Design review of the part built by this model. Coordinates are the model's own, in mm. Face numbers are marked on the shaded views. A direction names the side the tool comes from. Coordinates: 2 decimals unless noted, no trailing zeros. Write each loop counter-clockwise with the first axis right and the second up, starting at its lowest first coordinate (ties: lowest second). Pieces come first, ordered by that corner, then holes. Notation, with made-up numbers: (-28, 47) -> (22, 47) arc R15 ccw to (22, 69) -> close; hole circle Ø7 at (13, -22.5). An arc over 180 degrees is marked (long way). Write item = value, one per line. Start each with the question number.
Autodesk Inventor part; units mm, degrees
ref_plane "YZ Plane" through (0, 0, 0) normal (1, 0, 0) x (0, 1, 0)
ref_plane "XZ Plane" through (0, 0, 0) normal (0, 1, 0) x (-1, 0, 0)
ref_plane "XY Plane" through (0, 0, 0) normal (0, 0, 1) x (1, 0, 0)
sketch "Boceto3" plane through (0, 0, 0) normal (0, 0, 1) x (1, 0, 0)
  line L0 (-30, 8) -> (-30, -12)
  line L1 (-30, -22) -> (30, -22)
  line L2 (30, -12) -> (30, 8)
  arc A0 (-19.4936, 8) -> (19.4936, 8) centre (0, 22) ccw
  line L3 (-30, 8) -> (-19.4936, 8)
  line L4 (19.4936, 8) -> (30, 8)
  line L5 (-30, -22) -> (-70, -22)
  line L6 (-70, -22) -> (-70, -12)
  line L7 (-70, -12) -> (-30, -12)
  line L8 (30, -22) -> (70, -22)
  line L9 (70, -22) -> (70, -12)
  line L10 (70, -12) -> (30, -12)
  point P0 (0, 0)
  point P1 (0, -22)
  point P2 (30, 0)
  dimension "d16" = 60
  dimension "d38" = 24
  dimension "d39" = 10.5064
  dimension "d40" = 10.5064
  dimension "d41" = 30
  dimension "d42" = 30
  dimension "d43" = 22
  dimension "d44" = 40
  dimension "d45" = 10
  dimension "d46" = 40
  dimension "d47" = 10
extrude "Extrusión2" add sketch "Boceto3" along normal blind 9
sketch "Boceto5" plane through (0, 0, 9) normal (0, 0, 1) x (1, 0, 0)
  line L0 (-70, -22) -> (70, -22)
  line L1 (70, -22) -> (70, -12)
  line L2 (70, -12) -> (30, -12)
  line L3 (30, -12) -> (30, 8)
  line L4 (30, 8) -> (19.4936, 8)
  arc A0 (-19.4936, 8) -> (19.4936, 8) centre (0, 22) ccw
  line L5 (-19.4936, 8) -> (-30, 8)
  line L6 (-30, 8) -> (-30, -12)
  line L7 (-30, -12) -> (-70, -12)
  line L8 (-70, -12) -> (-70, -22)
  point P0 (0, 0)
  point P1 (-52.5, -17)
  point P2 (52.5, -17)
  dimension "d55" = 5
  dimension "d56" = 17.5
  dimension "d57" = 5
  dimension "d58" = 17.5
hole "Agujero2" at (-52.5, -17, 9) at (52.5, -17, 9) direction (0, 0, -1) diameter 5 depth 10 tip angle 118
sketch "Boceto6" plane through (-70, -22, 0) normal (0, -1, 0) x (1, 0, 0)
  line L0 (0, 0) -> (140, 0)
  line L1 (140, 0) -> (140, 9)
  line L2 (0, 9) -> (140, 9)
  line L3 (0, 0) -> (0, 9)
  line L4 (40, 0) -> (40, 9)
  line L5 (100, 0) -> (100, 9)
  point P0 (70, 0)
  point P1 (47.5, 4.5)
  point P2 (92.5, 4.5)
  dimension "d67" = 47.5
  dimension "d68" = 47.5
  dimension "d69" = 4.5
  dimension "d70" = 4.5
hole "Agujero3" at (-22.5, -22, 4.5) at (22.5, -22, 4.5) direction (0, 1, 0) diameter 5 depth 20 tip angle 118
properties part number "Soporte para Motor 2" material "Abedul"
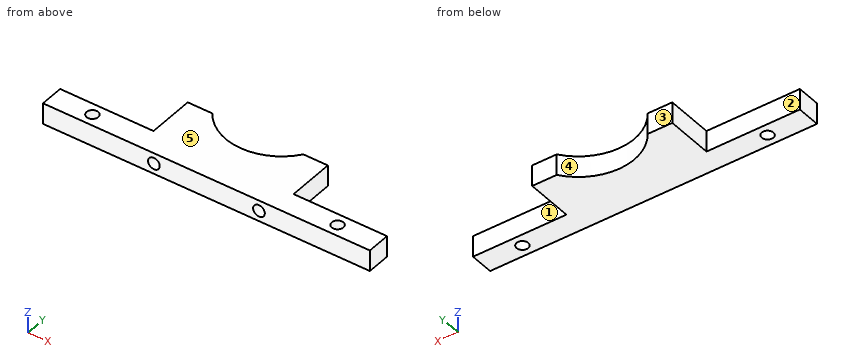
(1) Take a section at C-C, the plane y = -9.5. State the section outline as (x, z) points.
(2) For pin 1 Ø2.5 at (x, z) = (44, 5.5) entering from +Y, flat-tipped, find the tip position at first contact; note if it passes through.
(3) Take a section at D-D, the plane x = -12. State the section outline as (y, z) points, then the cut area to 3 significant figures.
(4) Take a section at A-A, the plane y = -17. State the section outline as (x, z) points, then the cut area to 3 significant figures.
(5) For the marked faces 1, 2 and 3, list the 3-axis set-ups (+Z, -Z, +X, -X, +Y, -Y) from which the entire face can be reached by the end or side of a thin tool; tool diameter is ignored.
(6) Take a section at B-B, the plane x = -52.5. State the section outline as (y, z) points.
(7) Mouldability with a two-part tool opening along X and no side actions: class the marked faces 4 and 5 as pulls with the +X half, pulls with the -X half, needs draft (parallel to the pull), parting line crosses it, or undercut.
(8) For line 1 (X direction, y = -11, z = 4.5), list the stretches that pass through material, from the lowest coordinate up.
Report:
q1.outline = (-30, 0) -> (30, 0) -> (30, 9) -> (-30, 9) -> close; hole circle Ø5 at (-22.5, 4.5); hole circle Ø5 at (22.5, 4.5)
q2.pin_1 = -12
q3.outline = (-22, 0) -> (1.22, 0) -> (1.22, 9) -> (-22, 9) -> close
q3.area = 209 mm2
q4.outline = (-70, 0) -> (-55, 0) -> (-55, 9) -> (-70, 9) -> close; (-50, 0) -> (50, 0) -> (50, 9) -> (-50, 9) -> close; (55, 0) -> (70, 0) -> (70, 9) -> (55, 9) -> close; hole circle Ø5 at (-22.5, 4.5); hole circle Ø5 at (22.5, 4.5)
q4.area = 1,130 mm2
q5.face_1 = +Z, -Z, +X, +Y
q5.face_2 = +Z, -Z, -X, +Y
q5.face_3 = +Z, -Z, +X, -X, +Y
q6.outline = (-22, 0) -> (-19.5, 0) -> (-19.5, 9) -> (-22, 9) -> close; (-14.5, 0) -> (-12, 0) -> (-12, 9) -> (-14.5, 9) -> close
q7.face_4 = undercut
q7.face_5 = needs draft
q8.line_1 = -30 to -25, -20 to 20, 25 to 30
